Verification items for the finished model (mm, model axes). Round coordinates to 2 decimals unless told otherwise and drop trailing zeros. Loops run counter-clockwise (first coordinate to the right, second up) from the corner with the lowest first, then second, coordinate; pieces in that order, holes last. Notation, with made-up numbers: (74.25, -2.5) -> (122.25, -2.5) arc R23 ccw to (122.25, 19.5) -> close; hole circle Ø11 at (82.25, 41). An arc over 180 degrees is marked (long way). Use a Markdown table: item, result. Add a question column.
```python
from build123d import *

# Parameters (mm, degrees)
F0_R     = 19.177
F0_R_2   = 17.526
F1_DEPTH = 38.1
F2_R     = 17.526
F3_DEPTH = 2.54
F4_R     = 6.35
F5_DEPTH = 25.4


with BuildPart() as f1:
    # F0 (on Front) → F1 (new body)
    with BuildSketch(Plane.XZ):
        Circle(F0_R)
        Circle(F0_R_2, mode=Mode.SUBTRACT)
    extrude(amount=-F1_DEPTH)

    # F2 (on Front) → F3 (join)
    with BuildSketch(Plane.XZ):
        Circle(F2_R)
    extrude(amount=-F3_DEPTH)

    # F4 (on face) → F5 (cut)
    with BuildSketch(Plane.XZ):
        Circle(F4_R)
    extrude(amount=-F5_DEPTH, mode=Mode.SUBTRACT)


solid = f1.part
```
1) Sectioned sample at C-C on y = 9. Enter the section's corners in (x, z).
2) Sectioned sample at A-A on x = 0. Enter the section's corners in (y, z), then the cut area to 3 significant figures.
3) Sectioned sample at D-D on z = -10. Enter the section's corners in (x, y).
4) Release check for a two-part mould opening along Z. For faces 1 (the face through (8, 2.54, 0)), 2 (the face through (8, 38.1, -16)), 3 (the face through (16.72, 20.07, 5.26)), 4 (the face through (-15.218, 18.783, -11.669)) record: released by +Z, released by -Z, zero draft, split by the parting line, or undercut.
5) Sectioned sample at B-B on z = 0. Enter the section's corners in (x, y), then the cut area to 3 significant figures.
6) Go/stop test with flat-tipped pins: pin 1 (12 mm diameter, centred on x = 12.5, y = 21.5, fed in from -Z); pin 2 (11.5 mm diameter, centred on x = 0, z = 0, fed in from -Y); pin 3 (6 mm diameter, centred on y = 13, z = -12.5, fed in from -X); pin 4 (3 mm diameter, centred on x = -8.5, y = 25, fed in from +Z). Record where each tip stops, or that it passes through.
7) Thickness scan on line 1 (Z direction, x = 0, y = 1); line 2 (Z direction, x = 0, y = 25); line 3 (Y direction, x = -17, z = 1). Record the ranges inside material, lowest first.
Geometry results:
| question | item | result |
|---|---|---|
| 1 | outline | circle Ø38.35 at (0, 0); hole circle Ø35.05 at (0, 0) |
| 2 | outline | (0, -19.18) -> (38.1, -19.18) -> (38.1, -17.53) -> (2.54, -17.53) -> (2.54, -6.35) -> (0, -6.35) -> close; (0, 6.35) -> (2.54, 6.35) -> (2.54, 17.53) -> (38.1, 17.53) -> (38.1, 19.18) -> (0, 19.18) -> close |
| 2 | area | 183 mm^2 |
| 3 | outline | (-16.36, 0) -> (16.36, 0) -> (16.36, 38.1) -> (14.39, 38.1) -> (14.39, 2.54) -> (-14.39, 2.54) -> (-14.39, 38.1) -> (-16.36, 38.1) -> close |
| 4 | face 1 | undercut |
| 4 | face 2 | zero draft |
| 4 | face 3 | undercut |
| 4 | face 4 | split by the parting line |
| 5 | outline | (-19.18, 0) -> (-6.35, 0) -> (-6.35, 2.54) -> (-17.53, 2.54) -> (-17.53, 38.1) -> (-19.18, 38.1) -> close; (6.35, 0) -> (19.18, 0) -> (19.18, 38.1) -> (17.53, 38.1) -> (17.53, 2.54) -> (6.35, 2.54) -> close |
| 5 | area | 183 mm^2 |
| 6 | pin 1 | z = -18.04 |
| 6 | pin 2 | through |
| 6 | pin 3 | x = -16.66 |
| 6 | pin 4 | z = 17.85 |
| 7 | line 1 | -19.18 to -6.35, 6.35 to 19.18 |
| 7 | line 2 | -19.18 to -17.53, 17.53 to 19.18 |
| 7 | line 3 | 0 to 2.54 |
